Read the model definition and answer for the solid it produces. Units are mm, in the model's axes. A direction names the side the tool comes from. Round coordinates to 2 decimals unless told otherwise and drop trailing zeros. Loops run counter-clockwise (first coordinate to the right, second up) from the corner with the lowest first, then second, coordinate; pieces in that order, holes last. Notation, with made-up numbers: M 85.25,70 L 142.25,70 A14 cw 142.25,78 Z; hole C -4.5,31 d9. An arc over 180 degrees is marked long. Write each question's results on one line, items separated by ' | '.
```python
from build123d import *

# Parameters (mm, degrees)
SKETCH1_W           = 106.662693993
SKETCH1_H           = 83.18856
SKETCH1_W_2         = 88.3
SKETCH1_H_2         = 42.78
BOSS_EXTRUDE1_DEPTH = 4
SKETCH1_4_W         = 88.3
SKETCH1_4_H         = 42.78
BOSS_EXTRUDE2_DEPTH = 6.35
SKETCH2_R           = 1.449406475
CUT_EXTRUDE1_DEPTH  = 86.959228837
BOSS_EXTRUDE3_DEPTH = 106.662693993
FILLET6_R           = 1
BOSS_EXTRUDE4_DEPTH = 2
FILLET7_R           = 1
SKETCH5_W           = 1.65
SKETCH5_H           = 33.3
CUT_EXTRUDE3_DEPTH  = 6.08
BOSS_EXTRUDE6_START = 1.5
SKETCH10_W          = 106.662693993
SKETCH10_H          = 93.062075056
SKETCH10_R          = 1.449406475
SKETCH10_W_2        = 88.3
SKETCH10_H_2        = 42.78
BOSS_EXTRUDE6_DEPTH = 1.5
BOSS_EXTRUDE7_DEPTH = 106.662693993
FILLET9_R           = 1
FILLET10_R          = 5


with BuildPart() as part:
    # Sketch1 → Boss-Extrude1 (new body)
    with BuildSketch(Plane(origin=(0, 0, 0), x_dir=(1, 0, 0), z_dir=(0, 1, 0))):
        with Locations((16.325985563, -8.370933327)):
            Rectangle(SKETCH1_W, SKETCH1_H)
        with Locations((15.929638567, -14.302731543)):
            Rectangle(SKETCH1_W_2, SKETCH1_H_2, mode=Mode.SUBTRACT)
    extrude(amount=BOSS_EXTRUDE1_DEPTH)

    # Sketch1<4> → Boss-Extrude2 (add)
    with BuildSketch(Plane(origin=(0, 0, 0), x_dir=(1, 0, 0), z_dir=(0, 1, 0))):
        Polygon((-33.005361433, -44.307731543), (65.60133256, -44.996613327), (65.60133256, 15.853526673), (-33.005361433, 15.702268457), align=None)
        with Locations((15.929638567, -14.302731543)):
            Rectangle(SKETCH1_4_W, SKETCH1_4_H, mode=Mode.SUBTRACT)
    extrude(amount=BOSS_EXTRUDE2_DEPTH)

    # Sketch2 → Cut-Extrude1 (cut, through all)
    with BuildSketch(Plane.XZ):
        with Locations(Location((9.192630415, -21.45022355, 0), (0, 0, 270))):
            Circle(SKETCH2_R)
    extrude(amount=-CUT_EXTRUDE1_DEPTH, mode=Mode.SUBTRACT)

    # Sketch3 → Boss-Extrude3 (add)
    with BuildSketch(Plane.ZY.offset(37.005361433)):
        Polygon((-32.832268457, 0), (-49.732268457, 0), (-46.932268457, 4), (-32.832268457, 4), align=None)
    extrude(amount=-BOSS_EXTRUDE3_DEPTH)

    # Fillet6
    fillet6_edges = [part.edges().sort_by_distance(p)[0] for p in [
        (-33.005361433, 6.35, 14.302731543),
        (16.297985564, 6.35, 44.652172435),
        (65.60133256, 6.35, 14.571543327),
        (16.297985564, 6.35, -15.777897565),
    ]]
    fillet(fillet6_edges, radius=FILLET6_R)

    # Sketch4 → Boss-Extrude4 (add)
    with BuildSketch(Plane(origin=(0, 4, 0), x_dir=(1, 0, 0), z_dir=(0, 1, 0))):
        with BuildLine():
            Line((64.864638567, 25.152939827), (-33.005361433, 25.152939827))
            ThreePointArc((-33.005361433, 25.152939827), (-34.005361433, 26.152939827), (-33.005361433, 27.152939827))
            Line((-33.005361433, 27.152939827), (64.864638567, 27.152939827))
            ThreePointArc((64.864638567, 27.152939827), (65.864638567, 26.152939827), (64.864638567, 25.152939827))
        make_face()
        with BuildLine():
            Line((-33.005361433, 41.932268457), (64.864638567, 41.932268457))
            ThreePointArc((64.864638567, 41.932268457), (65.864638567, 42.932268457), (64.864638567, 43.932268457))
            Line((64.864638567, 43.932268457), (-33.005361433, 43.932268457))
            ThreePointArc((-33.005361433, 43.932268457), (-34.005361433, 42.932268457), (-33.005361433, 41.932268457))
        make_face()
        with BuildLine():
            Line((64.864638567, -48.207731543), (-33.005361433, -48.207731543))
            ThreePointArc((-33.005361433, -48.207731543), (-34.005361433, -47.207731543), (-33.005361433, -46.207731543))
            Line((-33.005361433, -46.207731543), (64.864638567, -46.207731543))
            ThreePointArc((64.864638567, -46.207731543), (65.864638567, -47.207731543), (64.864638567, -48.207731543))
        make_face()
    extrude(amount=BOSS_EXTRUDE4_DEPTH)

    # Fillet7
    fillet7_edges = [part.edges().sort_by_distance(p)[0] for p in [
        (65.864638567, 6, -26.152939827),
        (15.929638567, 6, -27.152939827),
        (-34.005361433, 6, -26.152939827),
        (15.929638567, 6, -25.152939827),
        (65.864638567, 6, 47.207731543),
        (15.929638567, 6, 46.207731543),
        (-34.005361433, 6, 47.207731543),
        (15.929638567, 6, 48.207731543),
        (-34.005361433, 6, -42.932268457),
        (15.929638567, 6, -41.932268457),
        (65.864638567, 6, -42.932268457),
        (15.929638567, 6, -43.932268457),
    ]]
    fillet(fillet7_edges, radius=FILLET7_R - 0.0001)  # a hair under: the kernel refuses the full size

    # Sketch5 → Cut-Extrude3 (cut)
    with BuildSketch(Plane(origin=(0, 6.35, 0), x_dir=(1, 0, 0), z_dir=(0, 1, 0))):
        with Locations((-29.045361433, -14.302731543)):
            Rectangle(SKETCH5_W, SKETCH5_H)
    extrude(amount=-CUT_EXTRUDE3_DEPTH, mode=Mode.SUBTRACT)

    # Sketch10 → Boss-Extrude6 (add)
    with BuildSketch(Plane.XZ.offset(BOSS_EXTRUDE6_START)):
        with Locations((16.325985563, 3.434175799)):
            Rectangle(SKETCH10_W, SKETCH10_H)
        with Locations(Location((9.192630415, -21.45022355, 0), (0, 0, 270))):
            Circle(SKETCH10_R, mode=Mode.SUBTRACT)
        with Locations((15.929638567, 14.302731543)):
            Rectangle(SKETCH10_W_2, SKETCH10_H_2, mode=Mode.SUBTRACT)
    extrude(amount=-BOSS_EXTRUDE6_DEPTH)

    # Sketch11 → Boss-Extrude7 (add)
    with BuildSketch(Plane.ZY.offset(37.005361433)):
        Polygon((-49.732268457, 0), (-50.782268457, -1.5), (-43.096861729, -1.5), (-43.096861729, 0), align=None)
    extrude(amount=-BOSS_EXTRUDE7_DEPTH)

    # Fillet9
    fillet9_edges = [part.edges().sort_by_distance(p)[0] for p in [
        (9.192630415, -1.5, -20.000817075),
    ]]
    fillet(fillet9_edges, radius=FILLET9_R)

    # Fillet10
    fillet10_edges = [part.edges().sort_by_distance(p)[0] for p in [
        (-37.005361433, -1.5, -0.408527565),
        (69.65733256, -1.5, -0.408527565),
        (16.325985564, -1.5, 49.965213327),
    ]]
    fillet(fillet10_edges, radius=FILLET10_R)


solid = part.part
```
1. Which of the six approach directions +Z, -Z, +X, -X, +Y, -Y give full straight-line access (tool end or side, diameter ignored) to faces 5 (the face through (16.1, 6.35, -7.4)), 6 (the face through (-29.87, 3, 15)), 7 (the face through (15, 2, -7.087))?
Completed:
face 5: +Z, -Z, +X, -X, +Y | face 6: +Y | face 7: +Y, -Y
2. Find section A-A, the plane z = 4. Give the vertices of the cut face in (x, y), then the cut area to 3 significant figures.
Completed:
outline: M -37.01,3.5 A5 ccw -32.01,-1.5 L -28.22,-1.5 L -28.22,0.27 L -29.87,0.27 L -29.87,6.35 L -32.01,6.35 A1 ccw -33.01,5.35 L -33.01,4 L -37.01,4 Z; M 60.08,-1.5 L 64.66,-1.5 A5 ccw 69.66,3.5 L 69.66,4 L 65.6,4 L 65.6,5.35 A1 ccw 64.6,6.35 L 60.08,6.35 Z | area: 104 mm2
3. Given P1, Ø5, axis at x = 31, z = -30.5, coming from the +Y side; P2, Ø1.1, axis at x = 27.5, y = 4.5, coming from the -Z side; P3, Ø2.5, axis at x = 24.5, y = 3, coming from the -Z side, each flat-ended and moving along its own axis, determine where each tip first touches the part or whether it passes through.
Completed:
P1: stops at y = 4 | P2: stops at z = -46.97 | P3: stops at z = -48.51
4. Find section C-C, the plane z = 34.5. Give the vertices of the cut face in (x, y), then the cut area to 3 significant figures.
Completed:
outline: M -37.01,3.5 A5 ccw -32.01,-1.5 L -28.22,-1.5 L -28.22,6.35 L -32.01,6.35 A1 ccw -33.01,5.35 L -33.01,4 L -37.01,4 Z; M 60.08,-1.5 L 64.66,-1.5 A5 ccw 69.66,3.5 L 69.66,4 L 65.6,4 L 65.6,5.35 A1 ccw 64.6,6.35 L 60.08,6.35 Z | area: 114 mm2
5. Find section B-B, the plane z = -39.5. Give the vertices of the cut face in (x, y).
Completed:
outline: M -37.01,3.5 A5 ccw -32.01,-1.5 L 64.66,-1.5 A5 ccw 69.66,3.5 L 69.66,4 L -37.01,4 Z
6. Determine the mould class of faces 1 (the face through (15.58, 1.29, -48.83)), 2 (the face through (9.63, 1.72, -22.83)), 3 (the face through (17.073, -0.074, 48.462)), 4 (the face through (-35.502, -0.074, 0.297)) for opening direction Z: released by +Z, released by -Z, zero draft, split by the parting line, or undercut.
Completed:
face 1: released by -Z | face 2: undercut | face 3: released by +Z | face 4: zero draft
7. Find the intervals of material crossed by L1, parallel to Z at x = 64, y = 4.75; L2, parallel to Z at x = 42, y = 5; L3, parallel to Z at x = 1, y = 4.25, in increasing order.
Completed:
L1: z = -43.93 to -41.93, -27.15 to -25.15, -15.85 to 44.99, 46.21 to 48.21 | L2: z = -43.93 to -41.93, -27.15 to -25.15, -15.82 to -7.09, 35.69 to 44.83, 46.21 to 48.21 | L3: z = -43.93 to -41.93, -27.15 to -25.15, -15.75 to -7.09, 35.69 to 44.55, 46.21 to 48.21
